from build123d import *

# Parameters (mm, degrees)
EXTRUDE_1_DEPTH     = 190
SKETCH_2_R          = 2.25
CUT_EXTRUDE_1_DEPTH = 2
SKETCH_3_R          = 2.25
CUT_EXTRUDE_2_DEPTH = 2


with BuildPart() as part:
    # Эскиз1 → Бобышка-Вытянуть1 (new body)
    with BuildSketch(Plane(origin=(0, 0, 0), x_dir=(1, 0, 0), z_dir=(0, 1, 0))):
        Polygon((0, 0), (0, 20), (1, 20), (1, 1), (20, 1), (20, 0), align=None)
    extrude(amount=EXTRUDE_1_DEPTH)

    # Эскиз2 → Вырез-Вытянуть1 (cut, through all)
    with BuildSketch(Plane(origin=(1, 0, 0), x_dir=(0, 0, -1), z_dir=(1, 0, 0))):
        with Locations((10.5, 10)):
            Circle(SKETCH_2_R)
        with Locations((10.5, 180)):
            Circle(SKETCH_2_R)
    extrude(amount=-CUT_EXTRUDE_1_DEPTH, mode=Mode.SUBTRACT)

    # Эскиз3 → Вырез-Вытянуть2 (cut, through all)
    with BuildSketch(Plane(origin=(0, 0, -1), x_dir=(-1, 0, 0), z_dir=(0, 0, -1))):
        with Locations((-10.5, 180)):
            Circle(SKETCH_3_R)
        with Locations((-10.5, 10)):
            Circle(SKETCH_3_R)
    extrude(amount=-CUT_EXTRUDE_2_DEPTH, mode=Mode.SUBTRACT)


solid = part.part
Check sheet for the modelled part. Datum: model origin and axes. Units: mm. Give positions to 0.01 mm unless a question says otherwise; leave off trailing zeros. Order: outer loops, then holes, each group sorted by start corner. A loop starts at its lowest first (then second) coordinate and runs counter-clockwise, first axis right, second up. Notation, with made-up numbers: M 25.25,88 L 48.25,88 A19 ccw 48.25,111 Z; hole C 47,-24 d4. An arc over 180 degrees is marked long. Answer as CSV lines item,"result". Start each with the question number.
Item 1: Cross-section at D-D on y = 94.5. Enter the section's corners in (x, z).
Item 2: Mould release check, pull along X, two halves, no side actions. Record for faces 1 (the face through (1, 94, -11)), 2 (the face through (10, 94, -1)), 3 (the face through (10.988, 177.804, -0.507)): +X half, -X half, draft (parallel to the pull), parting line (faces both ways), or undercut.
Item 3: Gauge pin test, flat end, axial feed: P1, Ø10, axis at y = 84, z = -13, coming from the +X side. Record the tip position at first contact, or that the pin passes through.
Item 4: Cross-section at C-C on x = 10.5. Enter the section's corners in (y, z), plus the area to 3 significant figures.
Item 5: Cross-section at A-A on z = -10.5. Enter the section's corners in (x, y), plus the area to 3 significant figures.
Item 6: Cross-section at B-B on y = 10. Enter the section's corners in (x, z).
Item 7: Thickness scan on line 1 (Y direction, x = 10.5, z = -0.75); line 2 (Z direction, x = 4.25, y = 134.5); line 3 (X direction, y = 180, z = -0.4). Record the ranges inside material, lowest first. Write a range as [from, to].
Established:
1,outline,"M 0,-20 L 1,-20 L 1,-1 L 20,-1 L 20,0 L 0,0 Z"
2,face 1,"+X half"
2,face 2,"draft"
2,face 3,"undercut"
3,P1,"stops at x = 1"
4,outline,"M 0,-1 L 7.75,-1 L 7.75,0 L 0,0 Z; M 12.25,-1 L 177.75,-1 L 177.75,0 L 12.25,0 Z; M 182.25,-1 L 190,-1 L 190,0 L 182.25,0 Z"
4,area,"181 mm^2"
5,outline,"M 0,0 L 1,0 L 1,7.75 L 0,7.75 Z; M 0,12.25 L 1,12.25 L 1,177.75 L 0,177.75 Z; M 0,182.25 L 1,182.25 L 1,190 L 0,190 Z"
5,area,"181 mm^2"
6,outline,"M 0,-20 L 1,-20 L 1,-12.75 L 0,-12.75 Z; M 0,-8.25 L 1,-8.25 L 1,-1 L 8.25,-1 L 8.25,0 L 0,0 Z; M 12.75,-1 L 20,-1 L 20,0 L 12.75,0 Z"
7,line 1,"y = [0, 7.75], [12.25, 177.75], [182.25, 190]"
7,line 2,"z = [-1, 0]"
7,line 3,"x = [0, 8.25], [12.75, 20]"
